For this review, take the finished solid that the model builds, in its own axes (mm). Face numbers are marked on the shaded views. A direction names the side the tool comes from. Coordinates: 2 decimals unless noted, no trailing zeros. Write each loop counter-clockwise with the first axis right and the second up, starting at its lowest first coordinate (ties: lowest second). Pieces come first, ordered by that corner, then holes.
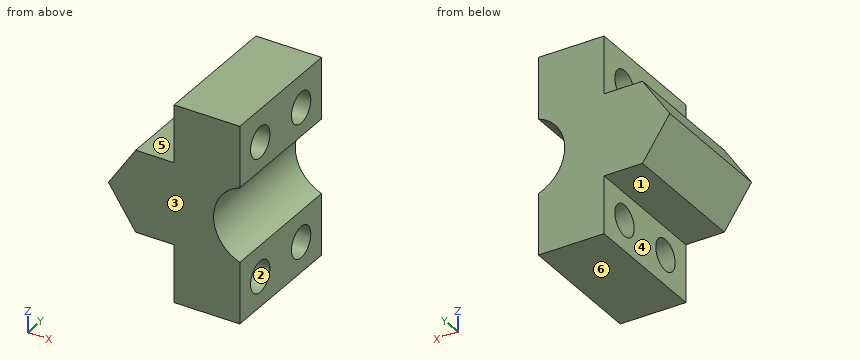
```python
from build123d import *

# Parameters (mm, degrees)
SKETCH1_W           = 12.7
SKETCH1_H           = 19.05
BOSS_EXTRUDE1_DEPTH = 12.7
CUT_EXTRUDE2_DEPTH  = 12.7
SKETCH5_R           = 1.5
CUT_EXTRUDE3_DEPTH  = 12.7
CUT_EXTRUDE4_DEPTH  = 12.7


with BuildPart() as part:
    # Sketch1 → Boss-Extrude1 (new body)
    with BuildSketch(Plane(origin=(0, 0, 0), x_dir=(1, 0, 0), z_dir=(0, 1, 0))):
        with Locations((6.35, 9.525)):
            Rectangle(SKETCH1_W, SKETCH1_H)
    extrude(amount=BOSS_EXTRUDE1_DEPTH)

    # Sketch4 → Cut-Extrude2 (cut)
    with BuildSketch(Plane(origin=(0, 12.7, 0), x_dir=(1, 0, 0), z_dir=(0, 1, 0))):
        Polygon((0, 19.05), (0, 9.525), (6.35, 19.05), align=None)
        Polygon((6.35, 0), (0, 9.525), (0, 0), align=None)
        with BuildLine():
            Line((12.7, 5.932897552), (12.7, 13.117102448))
            ThreePointArc((12.7, 13.117102448), (10.16, 9.525), (12.7, 5.932897552))
        make_face()
        with BuildLine():
            ThreePointArc((17.78, 9.525), (16.169704526, 12.635851973), (12.7, 13.117102448))
            Line((12.7, 13.117102448), (12.7, 5.932897552))
            ThreePointArc((12.7, 5.932897552), (16.169704526, 6.414148027), (17.78, 9.525))
        make_face()
    extrude(amount=-CUT_EXTRUDE2_DEPTH, mode=Mode.SUBTRACT)

    # Sketch5 → Cut-Extrude3 (cut)
    with BuildSketch(Plane(origin=(12.7, 0, 0), x_dir=(0, 0, -1), z_dir=(1, 0, 0))):
        with Locations((3.175, 9.525)):
            Circle(SKETCH5_R)
        with Locations((16.129, 9.525)):
            Circle(SKETCH5_R)
        with Locations((16.129, 3.175)):
            Circle(SKETCH5_R)
        with Locations((3.175, 3.175)):
            Circle(SKETCH5_R)
    extrude(amount=-CUT_EXTRUDE3_DEPTH, mode=Mode.SUBTRACT)

    # Sketch6 → Cut-Extrude4 (cut)
    with BuildSketch(Plane.XZ):
        Polygon((6.35, 0), (6.35, -5.570300529), (2.636466314, -5.570300529), align=None)
    cut_extrude4 = extrude(amount=-CUT_EXTRUDE4_DEPTH, mode=Mode.SUBTRACT)

    # Mirror1: Cut-Extrude4 across plane
    add(cut_extrude4.mirror(Plane(origin=(0, 0, -9.525), x_dir=(1, 0, 0), z_dir=(0, 0, -1))), mode=Mode.SUBTRACT)


solid = part.part
```
1) Tool access review of the marked faces 4, 5 and 6: name each direction out of +Z, -Z, +X, -X, +Y, -Y from which nothing blocks a thin tool from reaching the whole face with its end or side.
2) Clearance check with flat-ended pins moving along their axes: P1, Ø2, axis at x = 9, z = -7.5, coming from the -Y side; P2, Ø1, axis at x = 3.5, z = -4.5, coming from the -Y side; P3, Ø3, axis at y = 8.5, z = -17.5, coming from the -X side; P4, Ø1.1, axis at x = 4.5, y = 7, coming from the +Z side. State where each tip first meets the part, or that it passes through.
3) Consider section B-B (z = -3.5). Give the boundary of the cut face in (x, y), then the cut area to 4 significant figures.
4) The part is to be moulded in two halves that separate along Y. For the marked faces 1, 2 and 3, say which applies: pulls with the +Y half, pulls with the -Y half, needs draft (parallel to the pull), parting line crosses it, or undercut.
5) Consider section D-D (y = 10.5). Give the boundary of the cut face in (x, z) (3 decimals).
6) For L1, parallel to Y at x = 8, z = -16; L2, parallel to Y at x = 11.5, z = -16.5; L3, parallel to Z at x = 10, y = 9.75, list the stretches that pass through material, from the lowest coordinate up.
7) Consider section C-C (y = 7.5). Give the boundary of the cut face in (x, z) (3 decimals).
8) Consider section A-A (x = 11.25). Give the boundary of the cut face in (y, z) (3 decimals), then the cut area to 3 significant figures.
Results:
1. face 4: -Z, -X, +Y, -Y
1. face 5: +Z, -X, +Y, -Y
1. face 6: -Z, +X, -X, +Y, -Y
2. P1: stops at y = 0
2. P2: passes through
2. P3: stops at x = 6.35
2. P4: stops at z = -5.57
3. outline: (6.35, 0) - (12.7, 0) - (12.7, 1.71) - (6.35, 1.71) - close; (6.35, 4.64) - (12.7, 4.64) - (12.7, 8.06) - (6.35, 8.06) - close; (6.35, 10.99) - (12.7, 10.99) - (12.7, 12.7) - (6.35, 12.7) - close
3. area: 43.45 mm2
4. face 1: needs draft
4. face 2: undercut
4. face 3: pulls with the -Y half
5. outline: (0, -9.525) - (2.636, -13.48) - (6.35, -13.48) - (6.35, -14.989) - (12.7, -14.989) - (12.7, -13.117) arc R3.81 cw to (12.7, -5.933) - (12.7, -4.315) - (6.35, -4.315) - (6.35, -5.57) - (2.636, -5.57) - close; (6.35, -19.05) - (12.7, -19.05) - (12.7, -17.269) - (6.35, -17.269) - close; (6.35, -2.035) - (12.7, -2.035) - (12.7, 0) - (6.35, 0) - close
6. L1: y = 0 to 1.68, 4.67 to 8.03, 11.02 to 12.7
6. L2: y = 0 to 1.72, 4.63 to 8.07, 10.98 to 12.7
6. L3: z = -19.05 to -17.61, -14.65 to -4.66, -1.69 to 0
7. outline: (0, -9.525) - (2.636, -13.48) - (6.35, -13.48) - (6.35, -19.05) - (12.7, -19.05) - (12.7, -13.117) arc R3.81 cw to (12.7, -5.933) - (12.7, 0) - (6.35, 0) - (6.35, -5.57) - (2.636, -5.57) - close
8. outline: (0, -19.05) - (12.7, -19.05) - (12.7, -12.193) - (0, -12.193) - close; (0, -6.857) - (12.7, -6.857) - (12.7, 0) - (0, 0) - close; hole circle Ø3 at (3.175, -16.129); hole circle Ø3 at (3.175, -3.175); hole circle Ø3 at (9.525, -16.129); hole circle Ø3 at (9.525, -3.175)
8. area: 146 mm2
